```python
from build123d import *

# Parameters (mm, degrees)
F0_R     = 62
F1_DEPTH = 17
F2_R     = 60
F3_DEPTH = 15
F4_R     = 14.99999
F5_R     = 61
F5_R_2   = 60
F6_DEPTH = 4
F7_R     = 3.9
F8_DEPTH = 2
F9_DEPTH = 1
F10_D    = 3


# Not quite as in the source:
# - a fillet or chamfer is up to 0.001 mm smaller than in the source, because OpenCascade refuses the exact size


with BuildPart() as f1:
    # F0 (on Top) → F1 (new body)
    with BuildSketch(Plane.XY):
        Circle(F0_R)
    extrude(amount=-F1_DEPTH)

    # F2 (on face) → F3 (cut)
    with BuildSketch(Plane.XY):
        Circle(F2_R)
    extrude(amount=-F3_DEPTH, mode=Mode.SUBTRACT)

    # F4 (radius 15 in the source; OpenCascade refuses exactly that, so slightly less here)
    f4_edges = [f1.edges().sort_by_distance(p)[0] for p in [
        (-60, 0, -15),
        (-62, 0, -17),
    ]]
    fillet(f4_edges, radius=F4_R)

    # F5 (on face) → F6 (join)
    with BuildSketch(Plane.XY):
        Circle(F5_R)
        Circle(F5_R_2, mode=Mode.SUBTRACT)
    extrude(amount=F6_DEPTH)

    # F7 (on face) → F8 (join)
    with BuildSketch(Plane.XY.offset(-15)):
        Circle(F7_R)
        with BuildLine():
            ThreePointArc((2.6792506443, 1.1097819539), (2.8011848962, 0.7505752308), (2.875190098, 0.3785259574))
            ThreePointArc((2.875190098, 0.3785259574), (2.8937908774, 0.1896690748), (2.9, 0))
            ThreePointArc((2.9, 0), (2.8937908774, -0.1896690748), (2.875190098, -0.3785259574))
            ThreePointArc((2.875190098, -0.3785259574), (2.8011848962, -0.7505752308), (2.6792506443, -1.1097819539))
            ThreePointArc((2.6792506443, -1.1097819539), (2.511473671, -1.45), (2.3007246868, -1.7654081441))
            ThreePointArc((2.3007246868, -1.7654081441), (2.0506096654, -2.0506096654), (1.7654081441, -2.3007246868))
            ThreePointArc((1.7654081441, -2.3007246868), (1.45, -2.511473671), (1.1097819539, -2.6792506443))
            ThreePointArc((1.1097819539, -2.6792506443), (0.7505752308, -2.8011848962), (0.3785259574, -2.875190098))
            ThreePointArc((0.3785259574, -2.875190098), (0, -2.9), (-0.3785259574, -2.875190098))
            ThreePointArc((-0.3785259574, -2.875190098), (-0.7505752308, -2.8011848962), (-1.1097819539, -2.6792506443))
            ThreePointArc((-1.1097819539, -2.6792506443), (-1.45, -2.511473671), (-1.7654081441, -2.3007246868))
            ThreePointArc((-1.7654081441, -2.3007246868), (-2.0506096654, -2.0506096654), (-2.3007246868, -1.7654081441))
            ThreePointArc((-2.3007246868, -1.7654081441), (-2.511473671, -1.45), (-2.6792506443, -1.1097819539))
            ThreePointArc((-2.6792506443, -1.1097819539), (-2.8011848962, -0.7505752308), (-2.875190098, -0.3785259574))
            ThreePointArc((-2.875190098, -0.3785259574), (-2.9, 0), (-2.875190098, 0.3785259574))
            ThreePointArc((-2.875190098, 0.3785259574), (-2.8011848962, 0.7505752308), (-2.6792506443, 1.1097819539))
            ThreePointArc((-2.6792506443, 1.1097819539), (-2.511473671, 1.45), (-2.3007246868, 1.7654081441))
            ThreePointArc((-2.3007246868, 1.7654081441), (-2.0506096654, 2.0506096654), (-1.7654081441, 2.3007246868))
            ThreePointArc((-1.7654081441, 2.3007246868), (-1.45, 2.511473671), (-1.1097819539, 2.6792506443))
            ThreePointArc((-1.1097819539, 2.6792506443), (-0.7505752308, 2.8011848962), (-0.3785259574, 2.875190098))
            ThreePointArc((-0.3785259574, 2.875190098), (0, 2.9), (0.3785259574, 2.875190098))
            ThreePointArc((0.3785259574, 2.875190098), (0.7505752308, 2.8011848962), (1.1097819539, 2.6792506443))
            ThreePointArc((1.1097819539, 2.6792506443), (1.45, 2.511473671), (1.7654081441, 2.3007246868))
            ThreePointArc((1.7654081441, 2.3007246868), (2.0506096654, 2.0506096654), (2.3007246868, 1.7654081441))
            ThreePointArc((2.3007246868, 1.7654081441), (2.511473671, 1.45), (2.6792506443, 1.1097819539))
        make_face(mode=Mode.SUBTRACT)
        with BuildLine():
            Line((-2.6792506443, 1.1097819539), (-2.2170250337, 1.28))
            Line((-2.2170250337, 1.28), (-2.3007246868, 1.7654081441))
            ThreePointArc((-2.3007246868, 1.7654081441), (-2.511473671, 1.45), (-2.6792506443, 1.1097819539))
        make_face()
        with BuildLine():
            Line((-2.3007246868, 1.7654081441), (-1.8101933598, 1.8101933598))
            Line((-1.8101933598, 1.8101933598), (-1.7654081441, 2.3007246868))
            ThreePointArc((-1.7654081441, 2.3007246868), (-2.0506096654, 2.0506096654), (-2.3007246868, 1.7654081441))
        make_face()
        with BuildLine():
            Line((-1.7654081441, 2.3007246868), (-1.28, 2.2170250337))
            Line((-1.28, 2.2170250337), (-1.1097819539, 2.6792506443))
            ThreePointArc((-1.1097819539, 2.6792506443), (-1.45, 2.511473671), (-1.7654081441, 2.3007246868))
        make_face()
        with BuildLine():
            Line((-1.1097819539, 2.6792506443), (-0.6625767555, 2.4727701153))
            Line((-0.6625767555, 2.4727701153), (-0.3785259574, 2.875190098))
            ThreePointArc((-0.3785259574, 2.875190098), (-0.7505752308, 2.8011848962), (-1.1097819539, 2.6792506443))
        make_face()
        with BuildLine():
            Line((-0.3785259574, 2.875190098), (0, 2.56))
            Line((0, 2.56), (0.3785259574, 2.875190098))
            ThreePointArc((0.3785259574, 2.875190098), (0, 2.9), (-0.3785259574, 2.875190098))
        make_face()
        with BuildLine():
            Line((0.3785259574, 2.875190098), (0.6625767555, 2.4727701153))
            Line((0.6625767555, 2.4727701153), (1.1097819539, 2.6792506443))
            ThreePointArc((1.1097819539, 2.6792506443), (0.7505752308, 2.8011848962), (0.3785259574, 2.875190098))
        make_face()
        with BuildLine():
            Line((1.1097819539, 2.6792506443), (1.28, 2.2170250337))
            Line((1.28, 2.2170250337), (1.7654081441, 2.3007246868))
            ThreePointArc((1.7654081441, 2.3007246868), (1.45, 2.511473671), (1.1097819539, 2.6792506443))
        make_face()
        with BuildLine():
            Line((1.7654081441, 2.3007246868), (1.8101933598, 1.8101933598))
            Line((1.8101933598, 1.8101933598), (2.3007246868, 1.7654081441))
            ThreePointArc((2.3007246868, 1.7654081441), (2.0506096654, 2.0506096654), (1.7654081441, 2.3007246868))
        make_face()
        with BuildLine():
            Line((2.3007246868, 1.7654081441), (2.2170250337, 1.28))
            Line((2.2170250337, 1.28), (2.6792506443, 1.1097819539))
            ThreePointArc((2.6792506443, 1.1097819539), (2.511473671, 1.45), (2.3007246868, 1.7654081441))
        make_face()
        with BuildLine():
            Line((2.6792506443, 1.1097819539), (2.4727701153, 0.6625767555))
            Line((2.4727701153, 0.6625767555), (2.875190098, 0.3785259574))
            ThreePointArc((2.875190098, 0.3785259574), (2.8011848962, 0.7505752308), (2.6792506443, 1.1097819539))
        make_face()
        with BuildLine():
            ThreePointArc((2.9, 0), (2.8937908774, 0.1896690748), (2.875190098, 0.3785259574))
            Line((2.875190098, 0.3785259574), (2.56, 0))
            Line((2.56, 0), (2.875190098, -0.3785259574))
            ThreePointArc((2.875190098, -0.3785259574), (2.8937908774, -0.1896690748), (2.9, 0))
        make_face()
        with BuildLine():
            Line((2.875190098, -0.3785259574), (2.4727701153, -0.6625767555))
            Line((2.4727701153, -0.6625767555), (2.6792506443, -1.1097819539))
            ThreePointArc((2.6792506443, -1.1097819539), (2.8011848962, -0.7505752308), (2.875190098, -0.3785259574))
        make_face()
        with BuildLine():
            Line((2.6792506443, -1.1097819539), (2.2170250337, -1.28))
            Line((2.2170250337, -1.28), (2.3007246868, -1.7654081441))
            ThreePointArc((2.3007246868, -1.7654081441), (2.511473671, -1.45), (2.6792506443, -1.1097819539))
        make_face()
        with BuildLine():
            Line((2.3007246868, -1.7654081441), (1.8101933598, -1.8101933598))
            Line((1.8101933598, -1.8101933598), (1.7654081441, -2.3007246868))
            ThreePointArc((1.7654081441, -2.3007246868), (2.0506096654, -2.0506096654), (2.3007246868, -1.7654081441))
        make_face()
        with BuildLine():
            Line((1.7654081441, -2.3007246868), (1.28, -2.2170250337))
            Line((1.28, -2.2170250337), (1.1097819539, -2.6792506443))
            ThreePointArc((1.1097819539, -2.6792506443), (1.45, -2.511473671), (1.7654081441, -2.3007246868))
        make_face()
        with BuildLine():
            Line((-2.875190098, 0.3785259574), (-2.4727701153, 0.6625767555))
            Line((-2.4727701153, 0.6625767555), (-2.6792506443, 1.1097819539))
            ThreePointArc((-2.6792506443, 1.1097819539), (-2.8011848962, 0.7505752308), (-2.875190098, 0.3785259574))
        make_face()
        with BuildLine():
            Line((-2.875190098, -0.3785259574), (-2.56, 0))
            Line((-2.56, 0), (-2.875190098, 0.3785259574))
            ThreePointArc((-2.875190098, 0.3785259574), (-2.9, 0), (-2.875190098, -0.3785259574))
        make_face()
        with BuildLine():
            Line((-2.6792506443, -1.1097819539), (-2.4727701153, -0.6625767555))
            Line((-2.4727701153, -0.6625767555), (-2.875190098, -0.3785259574))
            ThreePointArc((-2.875190098, -0.3785259574), (-2.8011848962, -0.7505752308), (-2.6792506443, -1.1097819539))
        make_face()
        with BuildLine():
            Line((-2.3007246868, -1.7654081441), (-2.2170250337, -1.28))
            Line((-2.2170250337, -1.28), (-2.6792506443, -1.1097819539))
            ThreePointArc((-2.6792506443, -1.1097819539), (-2.511473671, -1.45), (-2.3007246868, -1.7654081441))
        make_face()
        with BuildLine():
            Line((-1.7654081441, -2.3007246868), (-1.8101933598, -1.8101933598))
            Line((-1.8101933598, -1.8101933598), (-2.3007246868, -1.7654081441))
            ThreePointArc((-2.3007246868, -1.7654081441), (-2.0506096654, -2.0506096654), (-1.7654081441, -2.3007246868))
        make_face()
        with BuildLine():
            Line((-1.1097819539, -2.6792506443), (-1.28, -2.2170250337))
            Line((-1.28, -2.2170250337), (-1.7654081441, -2.3007246868))
            ThreePointArc((-1.7654081441, -2.3007246868), (-1.45, -2.511473671), (-1.1097819539, -2.6792506443))
        make_face()
        with BuildLine():
            Line((-0.3785259574, -2.875190098), (-0.6625767555, -2.4727701153))
            Line((-0.6625767555, -2.4727701153), (-1.1097819539, -2.6792506443))
            ThreePointArc((-1.1097819539, -2.6792506443), (-0.7505752308, -2.8011848962), (-0.3785259574, -2.875190098))
        make_face()
        with BuildLine():
            Line((0.3785259574, -2.875190098), (0, -2.56))
            Line((0, -2.56), (-0.3785259574, -2.875190098))
            ThreePointArc((-0.3785259574, -2.875190098), (0, -2.9), (0.3785259574, -2.875190098))
        make_face()
        with BuildLine():
            Line((1.1097819539, -2.6792506443), (0.6625767555, -2.4727701153))
            Line((0.6625767555, -2.4727701153), (0.3785259574, -2.875190098))
            ThreePointArc((0.3785259574, -2.875190098), (0.7505752308, -2.8011848962), (1.1097819539, -2.6792506443))
        make_face()
    extrude(amount=F8_DEPTH)

    # F9 (cut): a face of the model
    f9_faces = [f1.faces().sort_by_distance(p)[0] for p in [
        (0, 0, -15),
    ]]
    extrude(f9_faces, amount=-F9_DEPTH, mode=Mode.SUBTRACT)

    # F10 (through all)
    with Locations(Plane.XY.offset(-15)):
        with Locations((0, 0)):
            Hole(F10_D / 2)


solid = f1.part
```
Verification items for the finished model (mm, model axes). A direction names the side the tool comes from. Coordinates: 2 decimals unless noted, no trailing zeros. Order: outer loops, then holes, each group sorted by start corner. A loop starts at its lowest first (then second) coordinate and runs counter-clockwise, first axis right, second up. Notation, with made-up numbers: (46, 9.5) -> (63, 9.5) arc R19 ccw to (63, 22.5) -> close; hole circle Ø8 at (30, 39). An arc over 180 degrees is marked (long way). Put each result on its own line as item: value. Start each with the question number.
1) Cross-section at B-B (z = -4). Enter the section's corners in (x, y).
2) Tool access check on faces 5 (the cylindrical face through (-59.94, 2.64, 1.97)), 6 (the cylindrical face through (1.5, 0.07, -16.51)). Record the directions out of +Z, -Z, +X, -X, +Y, -Y that give a thin tool (end or side, any length) a straight path to the whole face; none if there is none.
3) Go/stop test with flat-tipped pins: pin 1 (6 mm diameter, centred on x = -46.5, y = 29, fed in from -Z); pin 2 (4 mm diameter, centred on x = -34.5, z = -0.5, fed in from -Y); pin 3 (6.5 mm diameter, centred on x = 1, y = 0, fed in from +Z); pin 4 (2.5 mm diameter, centred on x = 0, y = 0, fed in from -Z). Record where each tip stops, or that it passes through.
4) Release check for a two-part mould opening along X. For faces 1 (the flat face through (-1, -10, -17)), 2 (the flat face through (0, 2, -16)), 3 (the cylindrical face through (-48.408, -37.118, 1.972)), 4 (the flat face through (-1, -9, -15)) record: pulls with the +X half, pulls with the -X half, needs draft (parallel to the pull), parting line crosses it, or undercut.
5) Cross-section at A-A (z = -10.5). Enter the section's corners in (x, y).
6) Material ranges on L1, parallel to Y at x = -1, z = 2.5; L2, parallel to Z at x = -5, y = -32; L3, parallel to X at y = -26, z = -7.5, recorded low to high.
Geometry check:
1. outline: circle Ø123.73 at (0, 0); hole circle Ø118.91 at (0, 0)
2. face 5: +Z
2. face 6: +Z, -Z
3. pin 1: stops at z = -16.21
3. pin 2: stops at y = -52.8
3. pin 3: stops at z = -13
3. pin 4: passes through
4. face 1: needs draft
4. face 2: undercut
4. face 3: parting line crosses it
4. face 4: undercut
5. outline: circle Ø118.72 at (0, 0); hole circle Ø111.42 at (0, 0)
6. L1: y = -60.99 to -59.99, 59.99 to 60.99
6. L2: z = -17 to -15
6. L3: x = -55.13 to -51.84, 51.84 to 55.13
